```python
from build123d import *

# Parameters (mm, degrees)
SKETCH_W      = 62.5
SKETCH_H      = 56.5
SKETCH_R      = 2.5
SKETCH_R_2    = 4
PAD_DEPTH     = 4
SKETCH001_R   = 20
SKETCH001_R_2 = 4
POCKET_DEPTH  = 1.5


with BuildPart() as part:
    # Sketch → Pad (new body)
    with BuildSketch(Plane.XY):
        Rectangle(SKETCH_W, SKETCH_H)
        with Locations((23.25, -23.25)):
            Circle(SKETCH_R, mode=Mode.SUBTRACT)
        with Locations((23.25, 23.25)):
            Circle(SKETCH_R, mode=Mode.SUBTRACT)
        with Locations((-23.25, 23.25)):
            Circle(SKETCH_R, mode=Mode.SUBTRACT)
        with Locations((-23.25, -23.25)):
            Circle(SKETCH_R, mode=Mode.SUBTRACT)
        Circle(SKETCH_R_2, mode=Mode.SUBTRACT)
    extrude(amount=PAD_DEPTH)

    # Sketch001 (on Face11 of Pad) → Pocket (cut)
    with BuildSketch(Plane.XY.offset(4)):
        Circle(SKETCH001_R)
        Circle(SKETCH001_R_2, mode=Mode.SUBTRACT)
    extrude(amount=-POCKET_DEPTH, mode=Mode.SUBTRACT)


solid = part.part
```
Verification items for the finished model (mm, model axes). A direction names the side the tool comes from. Coordinates: 2 decimals unless noted, no trailing zeros. Write each loop counter-clockwise with the first axis right and the second up, starting at its lowest first coordinate (ties: lowest second). Pieces come first, ordered by that corner, then holes. Notation, with made-up numbers: M 66.5,62.25 L 109.5,62.25 A27 cw 109.5,90.25 Z; hole C -28.5,34.5 d2. An arc over 180 degrees is marked long. Answer as a JSON object with one key per item and string values. Group by question number.
(1) Release check for a two-part mould opening along Y. For faces 1 (the face through (0, 28.25, 2)), 2 (the face through (7, 19, 4)), 3 (the face through (21.41, -21.56, 1.97)) record: +Y half, -Y half, draft (parallel to the pull), parting line (faces both ways), or undercut.
(2) Cross-section at A-A, the plane x = 0. Record the cut outline in (y, z).
(3) Tool access check on faces 4 (the face through (-4.336, -19.524, 3.26)), 5 (the face through (21.41, 24.94, 1.97)). Record the directions out of +Z, -Z, +X, -X, +Y, -Y that give a thin tool (end or side, any length) a straight path to the whole face; none if there is none.
(4) Gauge pin test, flat end, axial feed: pin 1 (4.5 mm diameter, centred on x = -23.25, y = 23.25, fed in from -Z). Record the tip position at first contact, or that the pin passes through.
(5) Cross-section at B-B, the plane y = 0. Record the cut outline in (x, z), and give its area (3 significant figures).
(6) Cross-section at D-D, the plane y = -23.25. Record the cut outline in (x, z).
(7) Cross-section at C-C, the plane x = 23.25. Record the cut outline in (y, z).
(8) Material ranges on line 1 (Y direction, x = -23.25, z = 2.75); line 2 (X direction, y = -23, z = 3.5); line 3 (X direction, y = -24, z = 2.45), recorded low to high.
Reply:
{
 "1": {"face 1": "+Y half", "face 2": "draft", "face 3": "undercut"},
 "2": {"outline": "M -28.25,0 L -4,0 L -4,2.5 L -20,2.5 L -20,4 L -28.25,4 Z; M 4,0 L 28.25,0 L 28.25,4 L 20,4 L 20,2.5 L 4,2.5 Z"},
 "3": {"face 4": "+Z", "face 5": "+Z, -Z"},
 "4": {"pin 1": "through"},
 "5": {"outline": "M -31.25,0 L -4,0 L -4,2.5 L -20,2.5 L -20,4 L -31.25,4 Z; M 4,0 L 31.25,0 L 31.25,4 L 20,4 L 20,2.5 L 4,2.5 Z", "area": "170 mm²"},
 "6": {"outline": "M -31.25,0 L -25.75,0 L -25.75,4 L -31.25,4 Z; M -20.75,0 L 20.75,0 L 20.75,4 L -20.75,4 Z; M 25.75,0 L 31.25,0 L 31.25,4 L 25.75,4 Z"},
 "7": {"outline": "M -28.25,0 L -25.75,0 L -25.75,4 L -28.25,4 Z; M -20.75,0 L 20.75,0 L 20.75,4 L -20.75,4 Z; M 25.75,0 L 28.25,0 L 28.25,4 L 25.75,4 Z"},
 "8": {"line 1": "-28.25 to -25.75, -20.75 to 20.75, 25.75 to 28.25", "line 2": "-31.25 to -25.74, -20.76 to 20.76, 25.74 to 31.25", "line 3": "-31.25 to -25.63, -20.87 to 20.87, 25.63 to 31.25"}
}
